Print and shaded views of the part. All mm, measured from the part's lowest x, y and z. A direction names the side the tool comes from. Round coordinates to 2 decimals unless told otherwise and drop trailing zeros. Loops run counter-clockwise (first coordinate to the right, second up) from the corner with the lowest first, then second, coordinate; pieces in that order, holes last. Notation, with made-up numbers: (-36, -14) - (-32, -14) arc R17 cw to (-32, 6) - close; hole circle Ø9 at (-11.5, 5). An arc over 180 degrees is marked (long way). Answer as a JSON object with one key per item and string values.
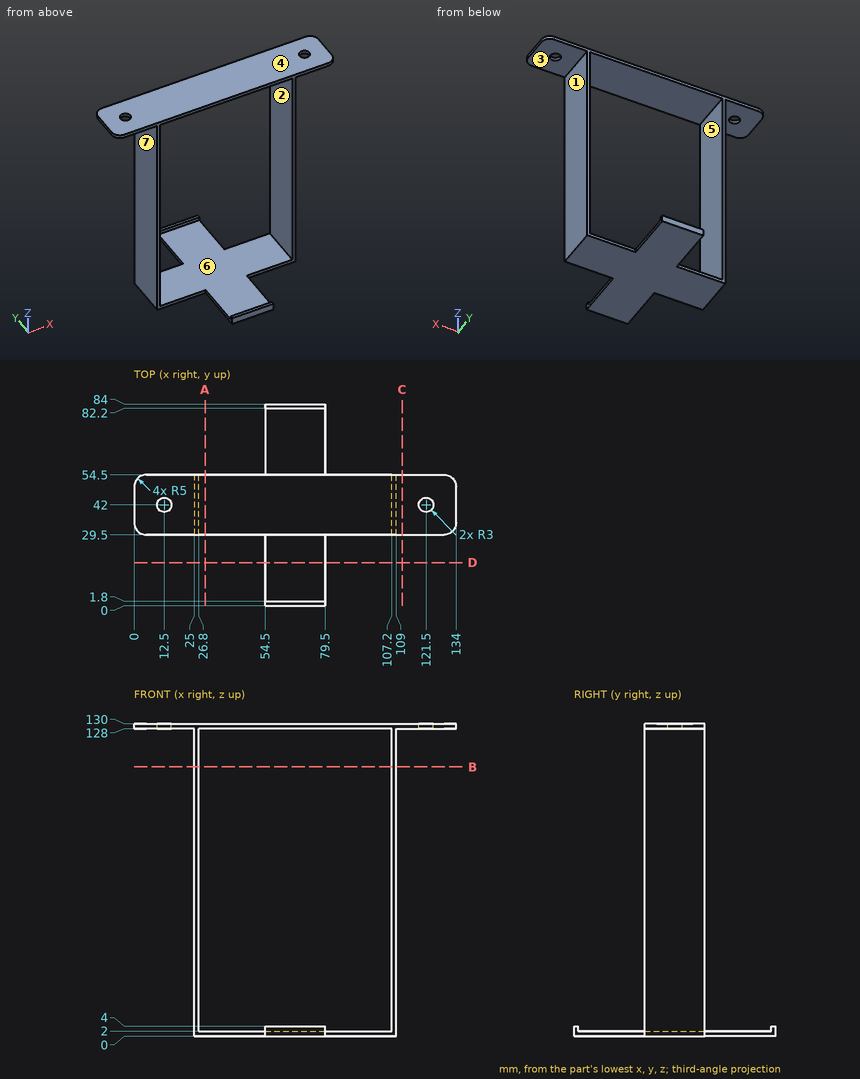
1) Probe probe 1 along X at (y, z) = (54, 13.5); probe 2 along Z at (x, y) = (52.5, 38); probe 3 along Z at (x, y) = (10, 51). List the from-to ranges inside material, lowest first.
Values follow:
{"probe 1": "25 to 26.8, 107.2 to 109", "probe 2": "0 to 2, 128 to 130", "probe 3": "128 to 130"}
2) Slice it at C-C on x = 111.5. List the corners of the cut face in (y, z).
Values follow:
{"outline": "(29.5, 128) - (54.5, 128) - (54.5, 130) - (29.5, 130) - close"}
3) Drop flat-ended pins along their axis: P1, Ø4.5, axis at y = 17, z = 2, coming from the -X side; P2, Ø7.5, axis at x = 16.5, y = 45.5, coming from the -Z side; P3, Ø12, axis at x = 84, y = 10.5, coming from the -Z side; P4, Ø2, axis at x = 62, y = 83.5, coming from the +Z side. Give the stop position or say it passes through.
Values follow:
{"P1": "x = 54.5", "P2": "z = 128", "P3": "z = 0", "P4": "z = 4"}
4) Tool access for the marked faces 4, 5, 6 and 7: list every direction of +Z, -Z, +X, -X, +Y, -Y with a clear straight run to the whole face (end or side of a thin tool).
Values follow:
{"face 4": "+Z, +X, -X, +Y, -Y", "face 5": "+Y, -Y", "face 6": "none", "face 7": "-Z, -X, +Y, -Y"}
5) Slice it at B-B on z = 112. List the corners of the cut face in (x, y), then the cut area to 3 significant figures.
Values follow:
{"outline": "(25, 29.5) - (26.8, 29.5) - (26.8, 54.5) - (25, 54.5) - close; (107.2, 29.5) - (109, 29.5) - (109, 54.5) - (107.2, 54.5) - close", "area": "90.0 mm²"}
6) Two-plate mould, pull along Z, no slides. Class the marked faces 1, 2 and 3: pulls with the +Z half, pulls with the -Z half, needs draft (parallel to the pull), parting line crosses it, or undercut.
Values follow:
{"face 1": "needs draft", "face 2": "undercut", "face 3": "pulls with the -Z half"}
7) Slice it at D-D on y = 18. List the corners of the cut face in (x, z).
Values follow:
{"outline": "(54.5, 0) - (79.5, 0) - (79.5, 2) - (54.5, 2) - close"}
8) Slice it at A-A on x = 29.5. List the corners of the cut face in (y, z), then the cut area to 3 significant figures.
Values follow:
{"outline": "(29.5, 0) - (54.5, 0) - (54.5, 2) - (29.5, 2) - close; (29.5, 128) - (54.5, 128) - (54.5, 130) - (29.5, 130) - close", "area": "100 mm²"}
